Print and shaded views of the part. All mm, measured from the part's lowest x, y and z. Give positions to 0.01 mm unless a question says otherwise; leave off trailing zeros. Write each loop counter-clockwise with the first axis right and the second up, starting at its lowest first coordinate (ties: lowest second). Pieces come first, ordered by that corner, then holes. Notation, with made-up numbers: (39.25, 53.25) -> (72.25, 53.25) arc R11 ccw to (72.25, 70.25) -> close; hole circle Ø4 at (6.25, 88.25). An arc over 180 degrees is marked (long way). Put each result on its own line as item: value.
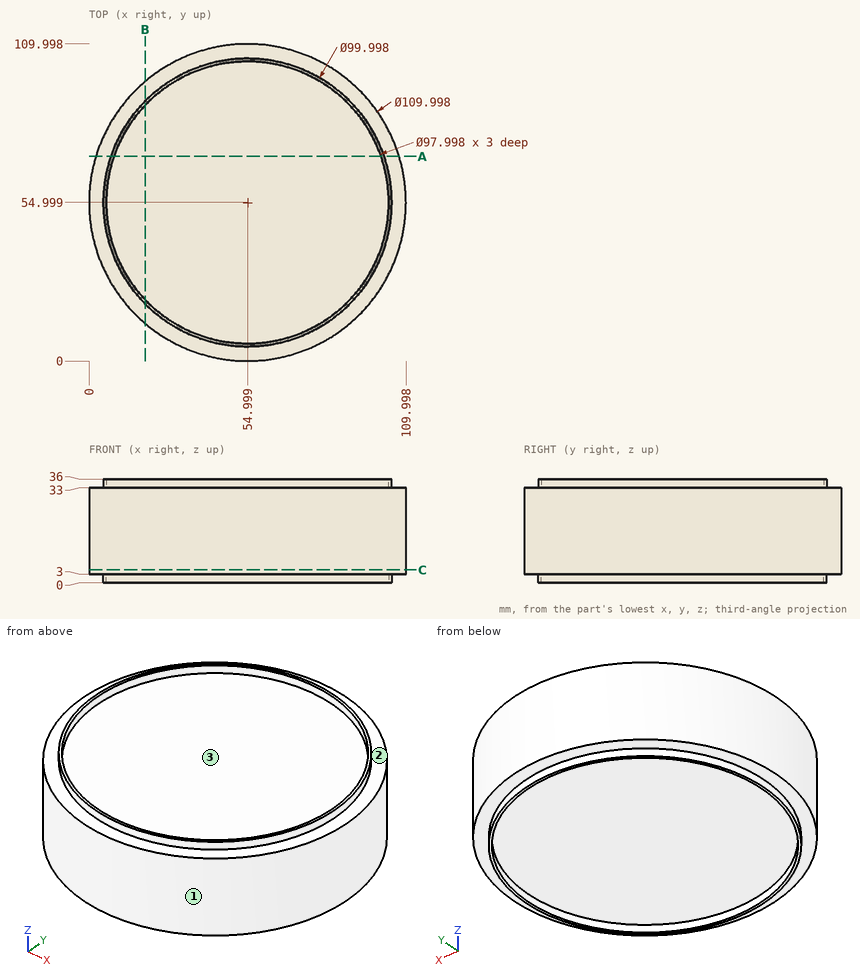
1) Pin check, flat tips, straight feed: pin 1 (8 mm diameter, centred on x = 27.5, y = 45.5, fed in from -Z); pin 2 (8 mm diameter, centred on y = 35.5, z = 12, fed in from +X); pin 3 (6 mm diameter, centred on x = 46.5, z = 26.5, fed in from -Y). Stop position of each tip, or through.
Filled sheet:
pin 1: z = 3
pin 2: x = 107.77
pin 3: y = 0.28
2) Slice it at C-C (z = 4.5). Write the cut outline in (x, y), plus the area to 3 significant figures.
Filled sheet:
outline: circle Ø110 at (55, 55)
area: 9,500 mm2
3) Pull direction X, two halves, no side cores. Call the marked faces 1, 2 and 3: released by +X, released by -X, zero draft, split by the parting line, or undercut.
Filled sheet:
face 1: split by the parting line
face 2: zero draft
face 3: undercut
4) Wall check: L1, parallel to Z at x = 67, y = 43.5; L2, parallel to X at y = 80, z = 9; L3, parallel to X at y = 64.5, z = 2. Give the ranges that are in metal, low to high.
Filled sheet:
L1: 3 to 33
L2: 6.01 to 103.99
L3: 5.91 to 6.93, 103.07 to 104.09
5) Slice it at A-A (y = 71). Write the cut outline in (x, z), plus the area to 3 significant figures.
Filled sheet:
outline: (2.38, 3) -> (7.63, 3) -> (7.63, 0) -> (8.69, 0) -> (8.69, 3) -> (101.31, 3) -> (101.31, 0) -> (102.37, 0) -> (102.37, 3) -> (107.62, 3) -> (107.62, 33) -> (102.37, 33) -> (102.37, 36) -> (101.31, 36) -> (101.31, 33) -> (8.69, 33) -> (8.69, 36) -> (7.63, 36) -> (7.63, 33) -> (2.38, 33) -> close
area: 3,170 mm2
6) Slice it at B-B (x = 19.5). Write the cut outline in (y, z).
Filled sheet:
outline: (12.99, 3) -> (19.79, 3) -> (19.79, 0) -> (21.22, 0) -> (21.22, 3) -> (88.77, 3) -> (88.77, 0) -> (90.21, 0) -> (90.21, 3) -> (97.01, 3) -> (97.01, 33) -> (90.21, 33) -> (90.21, 36) -> (88.77, 36) -> (88.77, 33) -> (21.22, 33) -> (21.22, 36) -> (19.79, 36) -> (19.79, 33) -> (12.99, 33) -> close
